Input: part model. Units: mm. Frame: model coordinates. Face numbers are marked on the shaded views. A direction names the side the tool comes from. Round coordinates to 2 decimals unless told otherwise and drop trailing zeros. Loops run counter-clockwise (first coordinate to the right, second up) from the corner with the lowest first, then second, coordinate; pieces in that order, holes last.
(1) First-contact query: pin 1 Ø3 at (x, y) = (44, 1.5) entering from +Z; pin 2 Ø0.9 at (x, z) = (42, -12.5) entering from +Y. Flat tips, straight axial feed; report the tip coordinate or a pass-through.
(2) Access query for the marked faces 4 and 5. Directions: +Z, -Z, +X, -X, +Y, -Y. A direction counts if a zero-diameter tool reaches every point of the face in a straight line with its end or side. Return the directions, or none.
(3) Line query: line 1 (Y direction, x = 41.1, z = -13.7); line 2 (Z direction, x = 42.75, y = 9.25); line 3 (Z direction, x = 43.35, y = 8). Output: solid intervals per line, ascending.
(4) Draft query along Z for the marked faces 1, 2 and 3. Return one class per face: released by +Z, released by -Z, zero draft, split by the parting line, or undercut.
(5) Cut plane A-A, the plane y = 7.75. Output: boundary loops of the cut face in (x, z), and give its area (3 significant figures).
(6) Cut plane B-B, the plane y = 1. Output: boundary loops of the cut face in (x, z).
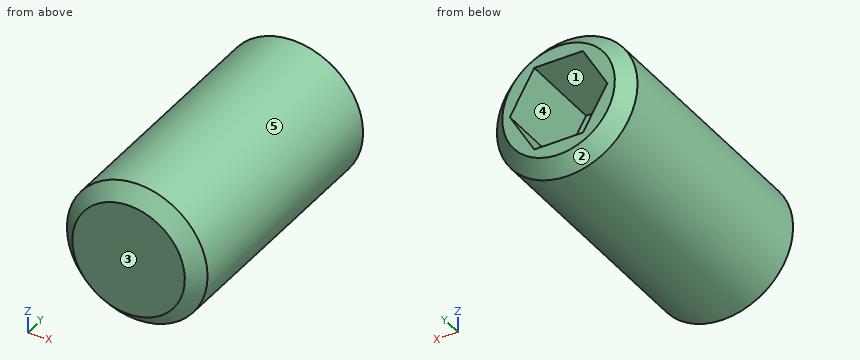
from build123d import *

# Parameters (mm, degrees)
SZKIC1_R                    = 2.5
DODANIE_WYCI_GNI_CIE1_DEPTH = 10
WYTNIJ_WYCI_GNI_CIE1_DEPTH  = 3
SFAZOWANIE1_SIZE            = 0.5


with BuildPart() as part:
    # Szkic1 → Dodanie-wyciągnięcie1 (new body)
    with BuildSketch(Plane(origin=(0, 0, 0), x_dir=(1, 0, 0), z_dir=(0, 1, 0))):
        with Locations(Location((42.20752559, 13.113324094, 0), (0, 0, 270))):
            Circle(SZKIC1_R)
    extrude(amount=DODANIE_WYCI_GNI_CIE1_DEPTH)

    # Szkic2 → Wytnij-wyciągnięcie1 (cut)
    with BuildSketch(Plane(origin=(0, 10, 0), x_dir=(1, 0, 0), z_dir=(0, 1, 0))):
        Polygon((43.939576398, 13.113324094), (43.073550994, 14.613324094), (41.341500186, 14.613324094), (40.475474782, 13.113324094), (41.341500186, 11.613324094), (43.073550994, 11.613324094), align=None)
    extrude(amount=-WYTNIJ_WYCI_GNI_CIE1_DEPTH, mode=Mode.SUBTRACT)

    # Sfazowanie1
    sfazowanie1_edges = [part.edges().sort_by_distance(p)[0] for p in [
        (42.20752559, 0, -15.613324094),
        (42.20752559, 10, -15.613324094),
    ]]
    chamfer(sfazowanie1_edges, length=SFAZOWANIE1_SIZE)


solid = part.part
Reported:
1. pin 1: stops at z = -10.63
1. pin 2: stops at y = 7
2. face 4: +Y
2. face 5: +Y, -Y
3. line 1: y = 0 to 7
3. line 2: z = -15.55 to -14.61, -11.61 to -10.67
3. line 3: z = -15.34 to -14.13, -12.09 to -10.89
4. face 1: undercut
4. face 2: split by the parting line
4. face 3: zero draft
5. outline: circle Ø5 at (42.21, -13.11); hole (40.48, -13.11) - (41.34, -14.61) - (43.07, -14.61) - (43.94, -13.11) - (43.07, -11.61) - (41.34, -11.61) - close
5. area: 11.8 mm2
6. outline: circle Ø5 at (42.21, -13.11)
